Check sheet for the drawn part. Datum: minimum x, y, z corner. Units: mm. Give positions to 0.01 mm unless a question says otherwise; leave off trailing zeros. Order: outer loops, then holes, each group sorted by start corner. A loop starts at its lowest first (then second) coordinate and runs counter-clockwise, first axis right, second up.
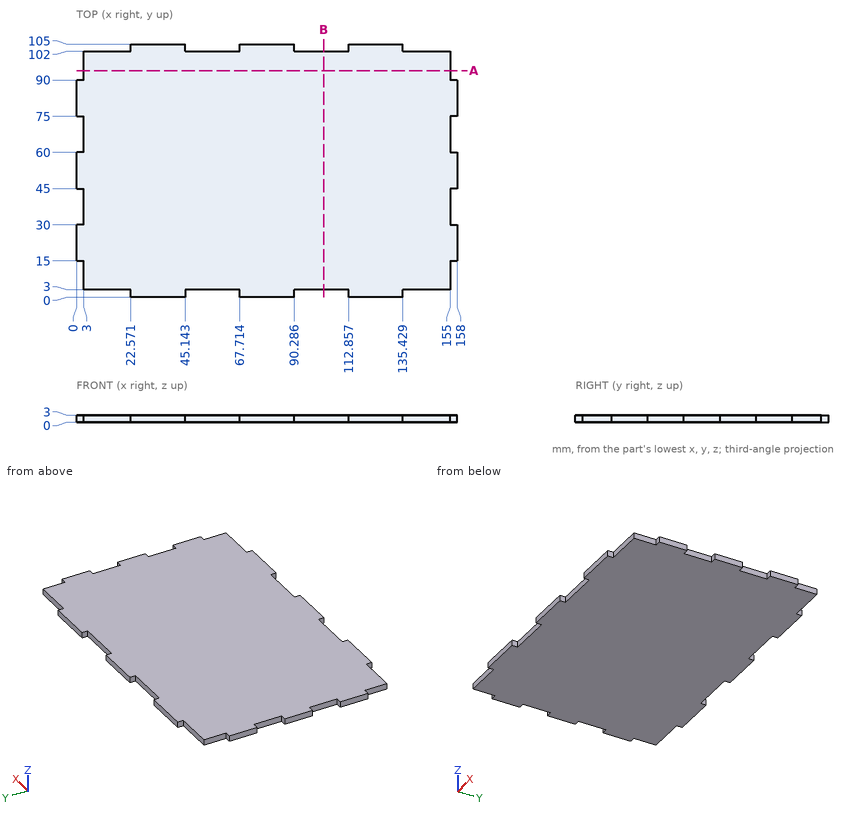
Item 1: Sectioned sample at A-A (y = 94). Enter the section's corners in (x, z), and give its area (3 significant figures).
Reported:
outline: (3, 0) - (155, 0) - (155, 3) - (3, 3) - close
area: 456 mm2
Item 2: Gauge pin test, flat ends, axial feed: pin 1 (0.9 mm diameter, centred on x = 1.5, z = 1, fed in from -Y); pin 2 (1.5 mm diameter, centred on x = 143.5, z = 1, fed in from -Y); pin 3 (1.5 mm diameter, centred on y = 9, z = 1, fed in from -X). Record the tip position at first contact, or that the pin passes through.
Reported:
pin 1: stops at y = 15
pin 2: stops at y = 3
pin 3: stops at x = 3
Item 3: Sectioned sample at B-B (x = 102.5). Enter the section's corners in (y, z).
Reported:
outline: (3, 0) - (102, 0) - (102, 3) - (3, 3) - close
Item 4: Scan lines: L1, parallel to Y at x = 51, z = 2.7; L2, parallel to X at y = 43, z = 2.6. Record each from-to range of solid material in increasing order.
Reported:
L1: y = 3 to 102
L2: x = 3 to 155
